Autodesk Fusion 360 part; units mm, degrees
sketch "Sketch1" plane through (0, 0, 0) normal (1, 0, 0) x (0, 1, 0)
  line L0 (0, 5) -> (3, 5)
  line L1 (3, 5) -> (3, 4.8)
  line L2 (3, 4.8) -> (1.5, 3.3)
  line L3 (1.5, 3.3) -> (1.5, 0.3)
  line L4 (1.2, 0) -> (0, 0)
  line L5 (0, 0) -> (0, 5)
  line L6 (1.5, 0.3) -> (1.2, 0)
  point P0 (1.5, 0)
  dimension "d1" = 1.5
  dimension "d3" = 5
  dimension "d4" = 1.7
  dimension "d5" = 135
  dimension "d6" = 3
  dimension "d9" = 0.3
  dimension "d10" = 0.3
revolve "Revolve1" add sketch "Sketch1" angle 360 about axis through (0, 0, 0) along (0, 0, 1)
sketch "Sketch2" plane through (0, 0, 5) normal (0, 0, 1) x (-1, 0, 0)
  circle A0 centre (0, 0) radius 3
  line L0 (0.5774, -1) -> (1.1547, 0)
  line L1 (1.1547, 0) -> (0.5774, 1)
  line L2 (0.5774, 1) -> (-0.5774, 1)
  line L3 (-0.5774, 1) -> (-1.1547, 0)
  line L4 (-1.1547, 0) -> (-0.5774, -1)
  line L5 (-0.5774, -1) -> (0.5774, -1)
  dimension "d11" = 1
extrude "Extrude1" cut sketch "Sketch2" against normal blind 1 contours L0 L1 L2 L3 L4 L5
equation "d1 = ( 3 / 2 ) * 1 mm"
equation "d3 = Length"
equation "d4 = Head_Length"
equation "d6 = Head_Diameter / 2"
equation "Length = 5 mm"
equation "d10 = d9"
equation "Head_Diameter = 6 mm"
equation "Head_Length = 1.7 mm"
properties part number "M3x5mm FHCS"
Here's how the part is built. I have some questions about the finished solid (model axes, mm). A direction names the side the tool comes from. Round coordinates to 2 decimals unless told otherwise and drop trailing zeros. Loops run counter-clockwise (first coordinate to the right, second up) from the corner with the lowest first, then second, coordinate; pieces in that order, holes last. Notation, with made-up numbers: (-17.5, 39) -> (0.5, 39) arc R21 ccw to (0.5, 63) -> close; hole circle Ø1 at (44.25, 47.25). An arc over 180 degrees is marked (long way). Write each question's results on one line, items separated by ' | '.
(1) For P1, Ø3, axis at x = -2, z = 0.5, coming from the +Y side; P2, Ø0.5, axis at x = 0, z = 4.5, coming from the -Y side; P3, Ø3, axis at y = 2.5, z = 1.5, coming from the -X side, each with a flat end and sliding along its axis, tell me the tip position at first contact or that it passes through.
Worked answers:
P1: y = 1.41 | P2: y = -2.95 | P3: x = -1.12
(2) If we section it at B-B, the plane z = 2.4: List the corners of the cut face in (x, y) for me.
Worked answers:
outline: circle Ø3 at (0, 0)
(3) If we section it at A-A, the plane x = 0: List the corners of the cut face in (y, z) for me, then the cut area to 3 significant figures.
Worked answers:
outline: (-3, 4.8) -> (-1.5, 3.3) -> (-1.5, 0.3) -> (-1.2, 0) -> (1.2, 0) -> (1.5, 0.3) -> (1.5, 3.3) -> (3, 4.8) -> (3, 5) -> (1, 5) -> (1, 4) -> (-1, 4) -> (-1, 5) -> (-3, 5) -> close | area: 15.8 mm2
(4) For faces 4 (the face through (0, 1.3, 5)), 5 (the face through (0.86, -0.51, 4.51)), which set-ups out of +Z, -Z, +X, -X, +Y, -Y let a thin tool reach every point of the face, with its end or its side?
Worked answers:
face 4: +Z, +X, -X, +Y, -Y | face 5: +Z
(5) If I drill on L1, parallel to Z at x = -0.3, y = 0.3; L2, parallel to Y at x = -0.8, z = 1.05; L3, parallel to Y at x = 0.25, z = 0.2, over which ranges is the centre line in solid material (lowest first)?
Worked answers:
L1: 0 to 4 | L2: -1.27 to 1.27 | L3: -1.38 to 1.38
(6) We'd pull the mould along X, two halves only. Please class faces 1 (the face through (0.07, -1.5, 1.78)), 2 (the face through (0, 0, 0)), 3 (the face through (0, -1, 4.5)): released by +X, released by -X, zero draft, split by the parting line, or undercut.
Worked answers:
face 1: split by the parting line | face 2: zero draft | face 3: undercut
